from build123d import *

# Parameters (mm, degrees)
F0_W     = 41
F0_H     = 106
F0_R     = 6
F0_R_2   = 2
F0_W_2   = 2.5
F0_H_2   = 14
F0_R_3   = 9.5
F1_DEPTH = 2
F2_R     = 2
F3_DEPTH = 14
F4_R     = 6.99999
F5_R     = 2.5
F6_DEPTH = 25


# Not quite as in the source:
# - a fillet or chamfer is up to 0.001 mm smaller than in the source, because OpenCascade refuses the exact size


with BuildPart() as f1:
    # F0 (on Top) → F1 (new body)
    with BuildSketch(Plane.XY):
        with Locations((0, 4.2499956787)):
            Rectangle(F0_W, F0_H)
        with Locations((-5.5959895056, -28.0965764523)):
            Circle(F0_R, mode=Mode.SUBTRACT)
        with Locations((-10.6551818848, -13.0636913106)):
            Circle(F0_R_2, mode=Mode.SUBTRACT)
        with Locations((-3, -7)):
            Rectangle(F0_W_2, F0_H_2, mode=Mode.SUBTRACT)
        with BuildLine():
            ThreePointArc((2, -23.0965764523), (-3.6071540429, -20.3211082876), (-6.5, -14.7736005353))
            Line((-6.5, -14.7736005353), (12.5, -15.1310515412))
            Line((12.5, -15.1310515412), (12.5, -41.1310515412))
            Line((12.5, -41.1310515412), (-6.5, -41.4195523692))
            ThreePointArc((-6.5, -41.4195523692), (-3.6071540429, -35.8720446169), (2, -33.0965764523))
            Line((2, -33.0965764523), (2, -23.0965764523))
        make_face(mode=Mode.SUBTRACT)
        with Locations((3, -7)):
            Rectangle(F0_W_2, F0_H_2, mode=Mode.SUBTRACT)
        with Locations((-10.6551818848, 5.2499956787)):
            Circle(F0_R_2, mode=Mode.SUBTRACT)
        with Locations((-10.6551818848, 23.5636826679)):
            Circle(F0_R_2, mode=Mode.SUBTRACT)
        with Locations((-5.5959895056, 38.5965678096)):
            Circle(F0_R, mode=Mode.SUBTRACT)
        with Locations((3.8262721598, 9.6499956787)):
            Circle(F0_R_3, mode=Mode.SUBTRACT)
        with BuildLine():
            ThreePointArc((2, 43.5965678096), (-3.6071540429, 46.3720359742), (-6.5, 51.9195437265))
            Line((-6.5, 51.9195437265), (12.5, 51.6310428985))
            Line((12.5, 51.6310428985), (12.5, 35.8656205144))
            Line((12.5, 35.8656205144), (14.3622287411, 31.5192815504))
            ThreePointArc((14.3622287411, 31.5192815504), (15.1282490927, 30.4976562448), (15.4, 29.2499956787))
            ThreePointArc((15.4, 29.2499956787), (14.5563858653, 27.1643303172), (12.5, 26.2516628086))
            Line((12.5, 26.2516628086), (12.5, 25.6310428985))
            Line((12.5, 25.6310428985), (-6.5, 25.2735918926))
            ThreePointArc((-6.5, 25.2735918926), (-3.6071540429, 30.8210996449), (2, 33.5965678096))
            Line((2, 33.5965678096), (2, 43.5965678096))
        make_face(mode=Mode.SUBTRACT)
    extrude(amount=F1_DEPTH)

    # F2
    f2_edges = [f1.edges().sort_by_distance(p)[0] for p in [
        (20.5, -48.750004, 1),
        (-20.5, -48.750004, 1),
        (12.5, -15.131052, 1),
        (12.5, -41.131052, 1),
        (12.5, 51.631043, 1),
        (20.5, 57.249996, 1),
        (-20.5, 57.249996, 1),
    ]]
    fillet(f2_edges, radius=F2_R)

    # F0 (on Top) → F3 (join)
    with BuildSketch(Plane.XY):
        with Locations((-3, -7)):
            Rectangle(F0_W_2, F0_H_2)
        with Locations((3, -7)):
            Rectangle(F0_W_2, F0_H_2)
    extrude(amount=F3_DEPTH)

    # F4 (radius 7 in the source; OpenCascade refuses exactly that, so slightly less here)
    f4_edges = [f1.edges().sort_by_distance(p)[0] for p in [
        (3, 0, 14),
        (3, -14, 14),
        (-3, -14, 14),
        (-3, 0, 14),
    ]]
    fillet(f4_edges, radius=F4_R)

    # F5 (on face) → F6 (cut)
    with BuildSketch(Plane.YZ.offset(4.25)):
        with Locations((-7, 8)):
            Circle(F5_R)
    extrude(amount=-F6_DEPTH, mode=Mode.SUBTRACT)


solid = f1.part
Can you work these out from the model? Positions are in its coordinate system, mm. A direction names the side the tool comes from. Round coordinates to 2 decimals unless told otherwise and drop trailing zeros. Order: outer loops, then holes, each group sorted by start corner. A loop starts at its lowest first (then second) coordinate and runs counter-clockwise, first axis right, second up. Notation, with made-up numbers: M 20,-1.5 L 49,-1.5 A22 cw 49,8.5 Z; hole C 20,-21 d7. An arc over 180 degrees is marked long. Use a Markdown table: item, result.
1) Imagine slicing it at B-B (y = -35.5). List the corners of the cut face in (x, z) for me, then the cut area to 3 significant figures.
Geometry says:
| item | result |
|---|---|
| outline | M -20.5,0 L -3.21,0 L -3.21,2 L -20.5,2 Z; M 12.5,0 L 20.5,0 L 20.5,2 L 12.5,2 Z |
| area | 50.6 mm² |
2) On a 3-axis mill with a long thin cutter (end or side, diameter ignored), from which of +Z, -Z, +X, -X, +Y, -Y can I reach the whole of each face in a straight line? I mean faces 4 (the face through (3, -14, 4)), 5 (the face through (-2.98, -5.85, 5.78)), 6 (the face through (1.75, -7, 5)), 7 (the face through (0, 57.25, 1)), 8 (the face through (13.42, 33.72, 0.99)). Say none if no direction works.
Geometry says:
| item | result |
|---|---|
| face 4 | +Z, +X, -X, -Y |
| face 5 | +X, -X |
| face 6 | +Z, +Y, -Y |
| face 7 | +Z, -Z, +X, -X, +Y |
| face 8 | +Z, -Z |
3) Imagine slicing it at C-C (z = 9). List the corners of the cut face in (x, y) for me, then the cut area to 3 significant figures.
Geometry says:
| item | result |
|---|---|
| outline | M -4.25,-13.71 L -1.75,-13.71 L -1.75,-9.29 L -4.25,-9.29 Z; M -4.25,-4.71 L -1.75,-4.71 L -1.75,-0.29 L -4.25,-0.29 Z; M 1.75,-13.71 L 4.25,-13.71 L 4.25,-9.29 L 1.75,-9.29 Z; M 1.75,-4.71 L 4.25,-4.71 L 4.25,-0.29 L 1.75,-0.29 Z |
| area | 44.2 mm² |
4) Imagine slicing it at A-A (z = 4). List the corners of the cut face in (x, y) for me, then the cut area to 3 significant figures.
Geometry says:
| item | result |
|---|---|
| outline | M -4.25,-14 L -1.75,-14 L -1.75,0 L -4.25,0 Z; M 1.75,-14 L 4.25,-14 L 4.25,0 L 1.75,0 Z |
| area | 70.0 mm² |
5) Imagine slicing it at D-D (y = -1.5). List the corners of the cut face in (x, z) for me.
Geometry says:
| item | result |
|---|---|
| outline | M -20.5,0 L 20.5,0 L 20.5,2 L 4.25,2 L 4.25,11.33 L 1.75,11.33 L 1.75,2 L -1.75,2 L -1.75,11.33 L -4.25,11.33 L -4.25,2 L -20.5,2 Z |
6) If I drill on line 1 along X through (y, z) = (-12, 4.5); line 2 along Y through (x, z) = (-3.5, 7); line 3 along Z through (x, y) = (-16, 15.5), over which ranges is the centre line in solid material (lowest first)?
Geometry says:
| item | result |
|---|---|
| line 1 | x = -4.25 to -1.75, 1.75 to 4.25 |
| line 2 | y = -14 to -9.29, -4.71 to 0 |
| line 3 | z = 0 to 2 |
7) I'm going to push flat-ended pins straight in: P1, Ø1.2, axis at x = 2.5, z = 4, coming from the +Y side; P2, Ø12.5, axis at x = 2, y = -17.5, coming from the +Z side; P3, Ø1, axis at y = -4.5, z = 9.5, coming from the +X side. Where does each tip first touch, or does it pass through?
Geometry says:
| item | result |
|---|---|
| P1 | stops at y = 0 |
| P2 | stops at z = 12.56 |
| P3 | stops at x = 4.25 |
8) If we mould it in two halves opening along X, with no side actions, what happens to faces 1 (the face through (-19.93, 56.65, 1.01)), 2 (the face through (20.5, 4, 1)), 3 (the face through (11.912, -15.678, 1.014))? For each: +X half, -X half, draft (parallel to the pull), parting line (faces both ways), or undercut.
Geometry says:
| item | result |
|---|---|
| face 1 | -X half |
| face 2 | +X half |
| face 3 | undercut |
